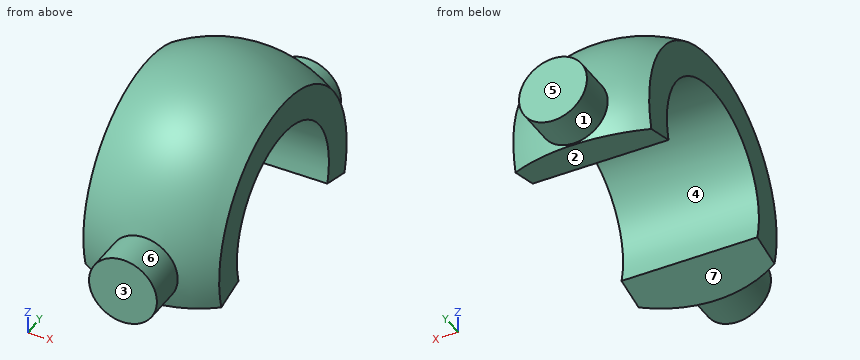
```python
from build123d import *

# Parameters (mm, degrees)
F1_ANGLE_BACK = 105
F1_ANGLE      = 210
F3_R          = 20


with BuildPart() as f1:
    # F0 (on Front) → F1 (revolve)
    with BuildSketch(Plane.XZ, mode=Mode.PRIVATE) as f1_sk:
        with BuildLine():
            ThreePointArc((40, 69.2820323028), (0, 80), (-40, 69.2820323028))
            Line((-40, 69.2820323028), (-40, 50))
            Line((-40, 50), (40, 50))
            Line((40, 50), (40, 69.2820323028))
        make_face()
    revolve(f1_sk.sketch.rotate(Axis((-190.0887642899, 0, 0), (-1, 0, 0)), -F1_ANGLE_BACK), axis=Axis((-190.0887642899, 0, 0), (-1, 0, 0)), revolution_arc=F1_ANGLE)

    # F3 (on offset) → F4 (join, up to the next surface of F1)
    with BuildSketch(Plane.XZ.offset(-100)):
        Circle(F3_R)
    extrude(until=Until.NEXT)

    # F5: F1 across plane


with BuildPart() as f1_1:
    add(f1.part)
    add(f1.part.mirror(Plane.XZ))


solid = f1_1.part
```
Geometry check sheet. Reference: the model listing, model coordinates, mm. Face numbers are marked on the shaded views. A direction names the side the tool comes from. Round coordinates to 2 decimals unless told otherwise and drop trailing zeros. Order: outer loops, then holes, each group sorted by start corner. A loop starts at its lowest first (then second) coordinate and runs counter-clockwise, first axis right, second up. Notation, with made-up numbers: M 46.25,81 L 62.25,81 A12 cw 62.25,103 Z; hole C -33.5,71 d2. An arc over 180 degrees is marked long. Write item = value, one per line.
Q1. Section check D-D (y = 43). Enter the section's corners in (x, z), plus the area to 3 significant figures.
Answer block:
outline = M -40,25.51 L 40,25.51 L 40,54.32 A67.46 ccw -40,54.32 Z
area = 3,020 mm^2
Q2. Section check A-A (z = 0). Enter the section's corners in (x, y), plus the area to 3 significant figures.
Answer block:
outline = M -40,-69.28 A80 ccw -20,-77.46 L -20,-100 L 20,-100 L 20,-77.46 A80 ccw 40,-69.28 L 40,-50 L -40,-50 Z; M -40,50 L 40,50 L 40,69.28 A80 ccw 20,77.46 L 20,100 L -20,100 L -20,77.46 A80 ccw -40,69.28 Z
area = 5,910 mm^2
Q3. Depth check by flat-ended pin: pin 1 Ø10 at (x, z) = (2, 70) entering from +Y; pin 2 Ø8 at (x, z) = (12, 43) entering from -Y; pin 3 Ø10 at (x, y) = (-17, -69) entering from -Z; pin 4 Ø8 at (y, z) = (26, 41.5) entering from +X. Enter the tip coordinate at first touch or a pass-through.
Answer block:
pin_1 = 46.6
pin_2 = -68.91
pin_3 = -19.83
pin_4 = 40
Q4. Section check B-B (x = 0). Enter the section's corners in (y, z), plus the area to 3 significant figures.
Answer block:
outline = M -100,-20 L -77.46,-20 A80 ccw -77.27,-20.71 L -48.3,-12.94 A50 cw long 48.3,-12.94 L 77.27,-20.71 A80 ccw 77.46,-20 L 100,-20 L 100,20 L 77.46,20 A80 ccw -77.46,20 L -100,20 Z
area = 8,810 mm^2
Q5. Scan lines: line 1 (Y direction, x = 5, z = 0); line 2 (Y direction, x = -25, z = 22.5); line 3 (Z direction, x = 15, y = 0). Record each from-to range of solid material in increasing order.
Answer block:
line_1 = -100 to -50, 50 to 100
line_2 = -72.59 to -44.65, 44.65 to 72.59
line_3 = 50 to 78.58
Q6. Section check C-C (z = 18). Enter the section's corners in (x, y).
Answer block:
outline = M -40,-66.9 A77.95 ccw -8.72,-77.46 L -8.72,-100 L 8.72,-100 L 8.72,-77.46 A77.95 ccw 40,-66.9 L 40,-46.65 L -40,-46.65 Z; M -40,46.65 L 40,46.65 L 40,66.9 A77.95 ccw 8.72,77.46 L 8.72,100 L -8.72,100 L -8.72,77.46 A77.95 ccw -40,66.9 Z
Q7. Release check for a two-part mould opening along Y. For the marked faces 4, 5, 6 and 7 record: released by +Y, released by -Y, zero draft, split by the parting line, or undercut.
Answer block:
face_4 = undercut
face_5 = released by +Y
face_6 = zero draft
face_7 = undercut
Q8. Set-up check for the marked faces 1, 2 and 3: record each of +Z, -Z, +X, -X, +Y, -Y from which the full face is reachable in a straight line by a thin tool's end or side.
Answer block:
face_1 = +Y
face_2 = -Z, +X, -X
face_3 = +Z, -Z, +X, -X, -Y
